The figure shows three views and two pictorial views of one solid part (mm, origin at its lowest corner). Answer the questions. A direction names the side the tool comes from. Round coordinates to 2 decimals unless told otherwise and drop trailing zeros. Loops run counter-clockwise (first coordinate to the right, second up) from the corner with the lowest first, then second, coordinate; pieces in that order, holes last. Notation, with made-up numbers: (44.25, 77) -> (87.25, 77) arc R16 cw to (87.25, 92) -> close; hole circle Ø5 at (-11.5, -32). An arc over 180 degrees is marked (long way). Write item = value, one per line. Start each with the question number.
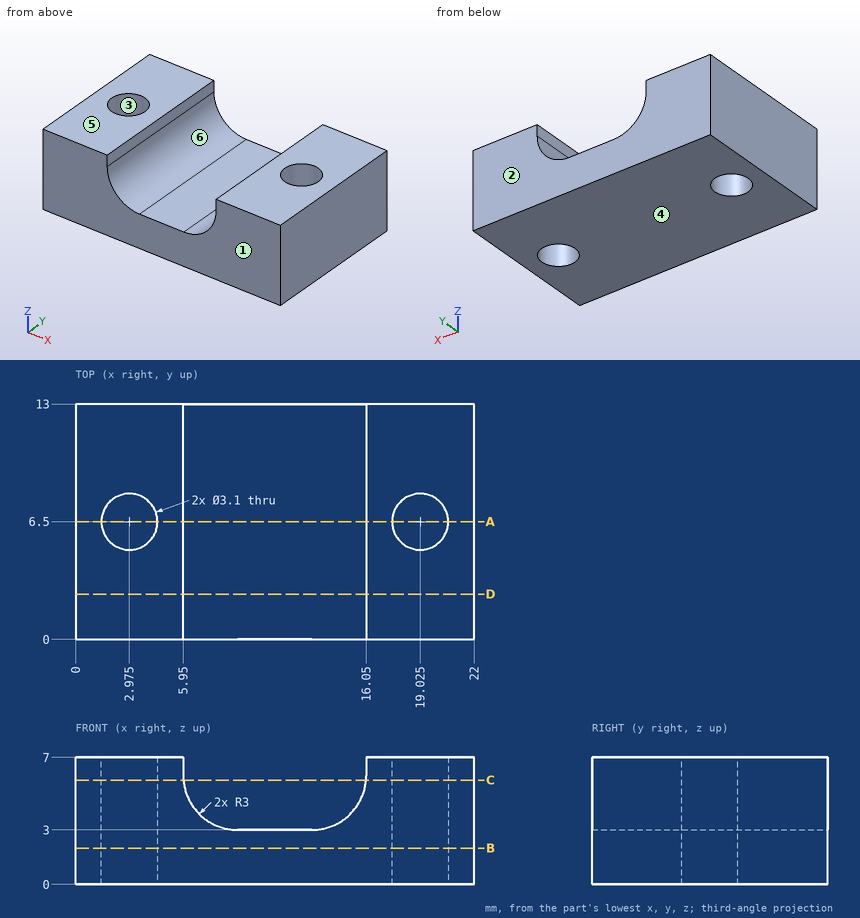
Item 1: Find the intervals of material crossed by line 1 along X through (y, z) = (7.5, 3.75); line 2 along X through (y, z) = (7, 1.5); line 3 along X through (y, z) = (5.5, 5.5), in increasing order. Write a range as [from, to].
Item 2: Section D-D (y = 2.5) is taken. Determine the outline of the cut face in (x, z).
Item 3: Section B-B (z = 2) is taken. Determine the outline of the cut face in (x, y) (3 decimals), then the cut area to 3 significant figures.
Item 4: The mould has two halves that part along Y. Classify the marked faces 1, 2, 3 and 4: pulls with the +Y half, pulls with the -Y half, needs draft (parallel to the pull), parting line crosses it, or undercut.
Item 5: Section A-A (y = 6.5) is taken. Determine the outline of the cut face in (x, z) (3 decimals).
Item 6: Section C-C (z = 5.75) is taken. Determine the outline of the cut face in (x, y) (3 decimals), then the cut area to 3 significant figures.
Item 7: Flat-ended cylindrical pins translate along their axes: pin 1 (6 mm diameter, centred on x = 11.5, y = 4.5, fed in from +Z); pin 2 (1.2 mm diameter, centred on x = 10.5, y = 7.5, fed in from +Z). Find the tip coordinate at first contact, or state that the pin passes through.
Item 8: A tool of negligible diameter and unlimited length cuts with its end or side. For the marked faces 5 and 6, from which of +Z, -Z, +X, -X, +Y, -Y can it reach the whole face along a straight path? Write none if from no direction.
Worked answers:
q1.line_1 = [0, 1.79], [4.16, 6.97], [15.03, 17.84], [20.21, 22]
q1.line_2 = [0, 1.51], [4.44, 17.56], [20.49, 22]
q1.line_3 = [0, 1.79], [4.16, 5.99], [16.01, 17.84], [20.21, 22]
q2.outline = (0, 0) -> (22, 0) -> (22, 7) -> (16.05, 7) -> (16.05, 6) arc R3 cw to (13.05, 3) -> (8.95, 3) arc R3 cw to (5.95, 6) -> (5.95, 7) -> (0, 7) -> close
q3.outline = (0, 0) -> (22, 0) -> (22, 13) -> (0, 13) -> close; hole circle Ø3.1 at (2.975, 6.5); hole circle Ø3.1 at (19.025, 6.5)
q3.area = 271 mm2
q4.face_1 = pulls with the -Y half
q4.face_2 = pulls with the +Y half
q4.face_3 = undercut
q4.face_4 = needs draft
q5.outline = (0, 0) -> (1.425, 0) -> (1.425, 7) -> (0, 7) -> close; (4.525, 0) -> (17.475, 0) -> (17.475, 7) -> (16.05, 7) -> (16.05, 6) arc R3 cw to (13.05, 3) -> (8.95, 3) arc R3 cw to (5.95, 6) -> (5.95, 7) -> (4.525, 7) -> close; (20.575, 0) -> (22, 0) -> (22, 7) -> (20.575, 7) -> close
q6.outline = (0, 0) -> (5.96, 0) -> (5.96, 13) -> (0, 13) -> close; (16.04, 0) -> (22, 0) -> (22, 13) -> (16.04, 13) -> close; hole circle Ø3.1 at (2.975, 6.5); hole circle Ø3.1 at (19.025, 6.5)
q6.area = 140 mm2
q7.pin_1 = 3.37
q7.pin_2 = 3
q8.face_5 = +Z, +X, -X, +Y, -Y
q8.face_6 = +Z, +Y, -Y
